```python
from build123d import *

# Parameters (mm, degrees)
SKETCH_1_R      = 1.249999998
SKETCH_1_R_2    = 1.25
EXTRUDE_1_DEPTH = 2
SKETCH_2_R      = 1.249999998
SKETCH_2_R_2    = 1.25
EXTRUDE_2_DEPTH = 2


with BuildPart() as part:
    # 草图1 → 凸台-拉伸1 (new body)
    with BuildSketch(Plane.XY):
        with BuildLine():
            Line((-6.26112666, -107.981945189), (-5.225850479, -104.118241884))
            ThreePointArc((-5.225850479, -104.118241884), (-4.973189102, -103.150666115), (-4.732884138, -102.17994774))
            ThreePointArc((-4.732884138, -102.17994774), (-4.069242074, -100.937454399), (-2.884606032, -100.175320593))
            ThreePointArc((-2.884606032, -100.175320593), (-1.923934791, -95.399938144), (-6.515491171, -97.026215112))
            ThreePointArc((-6.515491171, -97.026215112), (-7.154297104, -100.225141497), (-7.930442698, -103.393548202))
            Line((-7.930442698, -103.393548202), (-8.965718973, -107.257251863))
            ThreePointArc((-8.965718973, -107.257251863), (-28.541729969, -141.163897516), (-62.448375622, -160.739908512))
            Line((-62.448375622, -160.739908512), (-66.312078927, -161.775184692))
            ThreePointArc((-66.312078927, -161.775184692), (-105.464100918, -161.775184692), (-139.370746572, -142.199173697))
            Line((-139.370746572, -142.199173697), (-142.199173697, -139.370746572))
            ThreePointArc((-142.199173697, -139.370746572), (-161.775184692, -105.464100918), (-161.775184692, -66.312078927))
            Line((-161.775184692, -66.312078927), (-160.739908512, -62.448375622))
            ThreePointArc((-160.739908512, -62.448375622), (-141.163897516, -28.541729969), (-107.257251863, -8.965718973))
            Line((-107.257251863, -8.965718973), (-103.393548557, -7.930442793))
            ThreePointArc((-103.393548557, -7.930442793), (-100.225141676, -7.154297144), (-97.026215112, -6.515491171))
            ThreePointArc((-97.026215112, -6.515491171), (-95.399938144, -1.923934791), (-100.175320593, -2.884606032))
            ThreePointArc((-100.175320593, -2.884606032), (-100.937454399, -4.069242074), (-102.17994774, -4.732884138))
            ThreePointArc((-102.17994774, -4.732884138), (-103.150666115, -4.973189102), (-104.118241884, -5.225850479))
            Line((-104.118241884, -5.225850479), (-107.981945189, -6.26112666))
            ThreePointArc((-107.981945189, -6.26112666), (-124.151656982, -12.583052357), (-138.534502117, -22.307253601))
            ThreePointArc((-138.534502117, -22.307253601), (-140.602334013, -23.470064414), (-142.95588592, -23.768143523))
            ThreePointArc((-142.95588592, -23.768143523), (-145.123695491, -24.581931994), (-145.937483961, -26.749741565))
            ThreePointArc((-145.937483961, -26.749741565), (-146.235563071, -29.103293472), (-147.398373884, -31.171125368))
            ThreePointArc((-147.398373884, -31.171125368), (-157.122575127, -45.553970503), (-163.444500825, -61.723682296))
            Line((-163.444500825, -61.723682296), (-164.479777006, -65.587385601))
            ThreePointArc((-164.479777006, -65.587385601), (-167.089684647, -82.751729635), (-165.859701906, -100.069739522))
            ThreePointArc((-165.859701906, -100.069739522), (-165.88659415, -102.441939881), (-166.805226023, -104.629215177))
            ThreePointArc((-166.805226023, -104.629215177), (-167.184369319, -106.913487571), (-165.713885396, -108.702153845))
            ThreePointArc((-165.713885396, -108.702153845), (-163.824689209, -110.13707388), (-162.615299663, -112.178013531))
            ThreePointArc((-162.615299663, -112.178013531), (-155.02149102, -127.790841407), (-144.179072684, -141.350645559))
            Line((-144.179072684, -141.350645559), (-141.350645559, -144.179072684))
            ThreePointArc((-141.350645559, -144.179072684), (-127.790841407, -155.02149102), (-112.178013531, -162.615299663))
            ThreePointArc((-112.178013531, -162.615299663), (-110.13707388, -163.824689209), (-108.702153845, -165.713885396))
            ThreePointArc((-108.702153845, -165.713885396), (-106.913487571, -167.184369319), (-104.629215177, -166.805226023))
            ThreePointArc((-104.629215177, -166.805226023), (-102.441939881, -165.88659415), (-100.069739522, -165.859701906))
            ThreePointArc((-100.069739522, -165.859701906), (-82.751729635, -167.089684647), (-65.587385601, -164.479777006))
            Line((-65.587385601, -164.479777006), (-61.723682296, -163.444500825))
            ThreePointArc((-61.723682296, -163.444500825), (-45.553970503, -157.122575127), (-31.171125368, -147.398373884))
            ThreePointArc((-31.171125368, -147.398373884), (-29.103293472, -146.235563071), (-26.749741565, -145.937483961))
            ThreePointArc((-26.749741565, -145.937483961), (-24.581931994, -145.123695491), (-23.768143523, -142.95588592))
            ThreePointArc((-23.768143523, -142.95588592), (-23.470064414, -140.602334013), (-22.307253601, -138.534502117))
            ThreePointArc((-22.307253601, -138.534502117), (-12.583052357, -124.151656982), (-6.26112666, -107.981945189))
        make_face()
        with Locations((-97.515193216, -3.758518118)):
            Circle(SKETCH_1_R, mode=Mode.SUBTRACT)
        with Locations((-164.479777006, -106.188794245)):
            Circle(SKETCH_1_R_2, mode=Mode.SUBTRACT)
        with Locations((-106.188794245, -164.479777006)):
            Circle(SKETCH_1_R_2, mode=Mode.SUBTRACT)
        with Locations((-26.561830981, -143.143796504)):
            Circle(SKETCH_1_R_2, mode=Mode.SUBTRACT)
        with Locations((-3.758518118, -97.515193216)):
            Circle(SKETCH_1_R_2, mode=Mode.SUBTRACT)
        with Locations((-143.143796504, -26.561830981)):
            Circle(SKETCH_1_R_2, mode=Mode.SUBTRACT)
    extrude(amount=EXTRUDE_1_DEPTH)

    # 草图2 → 凸台-拉伸2 (add)
    with BuildSketch(Plane(origin=(0, 0, 0), x_dir=(-1, 0, 0), z_dir=(0, 0, -1))):
        with BuildLine():
            Line((4.259924653, -104.377060929), (5.295200833, -108.240764234))
            ThreePointArc((5.295200833, -108.240764234), (11.697726433, -124.616627957), (21.545904088, -139.182843786))
            ThreePointArc((21.545904088, -139.182843786), (22.520552994, -140.916066483), (22.770398003, -142.888774997))
            ThreePointArc((22.770398003, -142.888774997), (23.874825213, -145.830802272), (26.816852488, -146.935229482))
            ThreePointArc((26.816852488, -146.935229482), (28.789561001, -147.185074491), (30.522783699, -148.159723396))
            ThreePointArc((30.522783699, -148.159723396), (45.088999528, -158.007901052), (61.464863251, -164.410426652))
            Line((61.464863251, -164.410426652), (65.328566556, -165.445702832))
            ThreePointArc((65.328566556, -165.445702832), (82.711743348, -168.088884876), (100.250545121, -166.843220759))
            ThreePointArc((100.250545121, -166.843220759), (102.238884461, -166.865761396), (104.072222652, -167.635743529))
            ThreePointArc((104.072222652, -167.635743529), (107.172306616, -168.150295146), (109.599782274, -166.154638392))
            ThreePointArc((109.599782274, -166.154638392), (110.802508655, -164.571145209), (112.513190716, -163.557454775))
            ThreePointArc((112.513190716, -163.557454775), (128.325070661, -155.866830658), (142.05775234, -144.886179465))
            Line((142.05775234, -144.886179465), (144.886179465, -142.05775234))
            ThreePointArc((144.886179465, -142.05775234), (155.866830658, -128.325070661), (163.557454775, -112.513190716))
            ThreePointArc((163.557454775, -112.513190716), (164.571145209, -110.802508655), (166.154638392, -109.599782274))
            ThreePointArc((166.154638392, -109.599782274), (168.150295146, -107.172306616), (167.635743529, -104.072222652))
            ThreePointArc((167.635743529, -104.072222652), (166.865761396, -102.238884461), (166.843220759, -100.250545121))
            ThreePointArc((166.843220759, -100.250545121), (168.088884876, -82.711743348), (165.445702832, -65.328566556))
            Line((165.445702832, -65.328566556), (164.410426652, -61.464863251))
            ThreePointArc((164.410426652, -61.464863251), (158.007901052, -45.088999528), (148.159723396, -30.522783699))
            ThreePointArc((148.159723396, -30.522783699), (147.185074491, -28.789561001), (146.935229482, -26.816852488))
            ThreePointArc((146.935229482, -26.816852488), (145.830802272, -23.874825213), (142.888774997, -22.770398003))
            ThreePointArc((142.888774997, -22.770398003), (140.916066483, -22.520552994), (139.182843786, -21.545904088))
            ThreePointArc((139.182843786, -21.545904088), (124.616627957, -11.697726433), (108.240764234, -5.295200833))
            Line((108.240764234, -5.295200833), (104.377060933, -4.259924654))
            ThreePointArc((104.377060933, -4.259924654), (103.397149286, -4.00404203), (102.414054965, -3.760673355))
            ThreePointArc((102.414054965, -3.760673355), (101.615309246, -3.334046314), (101.125366085, -2.572494572))
            ThreePointArc((101.125366085, -2.572494572), (96.369116464, -0.135465803), (93.879703454, -4.864508258))
            ThreePointArc((93.879703454, -4.864508258), (94.48162483, -5.792369354), (95.484612817, -6.258470902))
            ThreePointArc((95.484612817, -6.258470902), (96.256077841, -6.382999122), (97.026215112, -6.515491171))
            ThreePointArc((97.026215112, -6.515491171), (100.225141676, -7.154297144), (103.393548557, -7.930442793))
            Line((103.393548557, -7.930442793), (107.257251863, -8.965718973))
            ThreePointArc((107.257251863, -8.965718973), (141.163897516, -28.541729969), (160.739908512, -62.448375622))
            Line((160.739908512, -62.448375622), (161.775184692, -66.312078927))
            ThreePointArc((161.775184692, -66.312078927), (161.775184692, -105.464100918), (142.199173697, -139.370746572))
            Line((142.199173697, -139.370746572), (139.370746572, -142.199173697))
            ThreePointArc((139.370746572, -142.199173697), (105.464100918, -161.775184692), (66.312078927, -161.775184692))
            Line((66.312078927, -161.775184692), (62.448375622, -160.739908512))
            ThreePointArc((62.448375622, -160.739908512), (28.541729969, -141.163897516), (8.965718973, -107.257251863))
            Line((8.965718973, -107.257251863), (7.930442698, -103.393548202))
            ThreePointArc((7.930442698, -103.393548202), (7.154297104, -100.225141497), (6.515491171, -97.026215112))
            ThreePointArc((6.515491171, -97.026215112), (6.382999122, -96.256077841), (6.258470902, -95.484612817))
            ThreePointArc((6.258470902, -95.484612817), (5.792369354, -94.48162483), (4.864508258, -93.879703454))
            ThreePointArc((4.864508258, -93.879703454), (0.135465803, -96.369116464), (2.572494572, -101.125366085))
            ThreePointArc((2.572494572, -101.125366085), (3.334046314, -101.615309246), (3.760673355, -102.414054965))
            ThreePointArc((3.760673355, -102.414054965), (4.004042029, -103.397149283), (4.259924653, -104.377060929))
        make_face()
        with Locations(Location((97.515193216, -3.758518118, 0), (0, 0, 180))):
            Circle(SKETCH_2_R, mode=Mode.SUBTRACT)
        with Locations(Location((164.479777006, -106.188794245, 0), (0, 0, 180))):
            Circle(SKETCH_2_R_2, mode=Mode.SUBTRACT)
        with Locations(Location((106.188794245, -164.479777006, 0), (0, 0, 180))):
            Circle(SKETCH_2_R_2, mode=Mode.SUBTRACT)
        with Locations(Location((26.561830981, -143.143796504, 0), (0, 0, 180))):
            Circle(SKETCH_2_R_2, mode=Mode.SUBTRACT)
        with Locations(Location((3.758518118, -97.515193216, 0), (0, 0, 180))):
            Circle(SKETCH_2_R_2, mode=Mode.SUBTRACT)
        with Locations(Location((143.143796504, -26.561830981, 0), (0, 0, 180))):
            Circle(SKETCH_2_R_2, mode=Mode.SUBTRACT)
    extrude(amount=-EXTRUDE_2_DEPTH)


solid = part.part
```
Design review of the part built by this model. Coordinates are the model's own, in mm. A direction names the side the tool comes from. Round coordinates to 2 decimals unless told otherwise and drop trailing zeros. Write each loop counter-clockwise with the first axis right and the second up, starting at its lowest first coordinate (ties: lowest second). Pieces come first, ordered by that corner, then holes.
Item 1: We need section A-A on x = -155.5. Write out the cut boundary in (y, z).
Item 2: For probe 1 along Y at (x, z) = (-96.5, 1.7); probe 2 along X at (y, z) = (-111, 0.6); probe 3 along Y at (x, z) = (-127, 0.9), list the stretches that pass through material, from the lowest coordinate up.
Item 3: We need section B-B on y = -115.5. Write out the cut boundary in (x, z).
Item 4: For faces 4 (the cylindrical face through (-28.15, -140.77, 0.99)), 5 (the cylindrical face through (-104.928, -161.917, 0.986)), 6 (the cylindrical face through (-141.555, -28.935, 0.986)), 7 (the cylindrical face through (-158.122, -45.308, 0.986)), list the 3-axis set-ups (+Z, -Z, +X, -X, +Y, -Y) from which the entire face can be reached by the end or side of a thin tool; tool diameter is ignored.
Item 5: Clearance check with flat-ended pins moving along their axes: pin 1 Ø3 at (x, y) = (-106.19, -164.48) entering from -Z; pin 2 Ø1 at (x, z) = (-140, 0.5) entering from +Y; pin 3 Ø2 at (x, y) = (-97.52, -3.76) entering from +Z. State where each tip first meets the part, or that it passes through.
Item 6: We need section C-C on z = 1. State how many separate pieces and enclosed holes the cut face has, and give its area (3 significant figures).
Item 7: We need section D-D on y = -36. Write out the cut boundary in (x, z), and give its area (3 significant figures).
Item 8: The part is to be moulded in two halves that separate along X. For faces 1 (the cylindrical face through (-161.63, -106, 0.99)), 2 (the cylindrical face through (-11.583, -124.398, 0.986)), 3 (the flat face through (-127.4, -152.3, 0)), say which applies: +X half, -X half, draft (parallel to the pull), parting line (faces both ways), or undercut.
Returned:
1. outline: (-128.9, 0) - (-121.4, 0) - (-121.4, 2) - (-128.9, 2) - close; (-48.54, 0) - (-40.66, 0) - (-40.66, 2) - (-48.54, 2) - close
2. probe 1: y = -167.44 to -163.6, -6.42 to -4.49, -3.03 to -0.1
2. probe 2: x = -164.4 to -160.06, -10.07 to -6.09
2. probe 3: y = -156.69 to -152.2, -17.41 to -13
3. outline: (-162.43, 0) - (-158.31, 0) - (-158.31, 2) - (-162.43, 2) - close; (-11.69, 0) - (-7.62, 0) - (-7.62, 2) - (-11.69, 2) - close
4. face 4: +Z, -Z, +Y
4. face 5: +Z, -Z
4. face 6: +Z, -Z, +X
4. face 7: +Z, -Z, -X, +Y
5. pin 1: stops at z = 0
5. pin 2: stops at y = -21.8
5. pin 3: passes through
6. separate pieces: 1
6. enclosed holes: 6
6. area: 1,460 mm2
7. outline: (-152.43, 0) - (-147.7, 0) - (-147.7, 2) - (-152.43, 2) - close
7. area: 9.45 mm2
8. face 1: undercut
8. face 2: +X half
8. face 3: draft
